Model file for the job. Use its own axes, mm. A direction names the side the tool comes from. Give positions to 0.01 mm unless a question says otherwise; leave off trailing zeros. Loops run counter-clockwise (first coordinate to the right, second up) from the corner with the lowest first, then second, coordinate; pieces in that order, holes last. Notation, with made-up numbers: M -30,21 L 10,21 A19 cw 10,33 Z; hole C 67,16.5 d4. An arc over 180 degrees is marked long. Answer in a Markdown table with one row per item.
```python
from build123d import *

# Parameters (mm, degrees)
F2_W      = 77
F2_H      = 64
F3_DEPTH  = 22
F4_W      = 73
F4_H      = 60
F5_DEPTH  = 20
F6_W      = 13
F6_H      = 12
F8_DEPTH  = 2
F7_W      = 12
F7_H      = 12
F9_DEPTH  = 2
F10_R     = 3.5
F11_DEPTH = 3


with BuildPart() as f3:
    # F2 (on Top) → F3 (new body)
    with BuildSketch(Plane.XY):
        with Locations((3.2737072408, 3.8249654726)):
            Rectangle(F2_W, F2_H)
    extrude(amount=F3_DEPTH)

    # F4 (on face) → F5 (cut)
    with BuildSketch(Plane.XY.offset(22)):
        with Locations((3.2737072408, 3.8249654726)):
            Rectangle(F4_W, F4_H)
    extrude(amount=-F5_DEPTH, mode=Mode.SUBTRACT)

    # F6 (on face) → F8 (cut)
    with BuildSketch(Plane.YZ.offset(41.7737072408)):
        with Locations((-9.3750345274, 12)):
            Rectangle(F6_W, F6_H)
    extrude(amount=-F8_DEPTH, mode=Mode.SUBTRACT)

    # F7 (on face) → F9 (cut)
    with BuildSketch(Plane.YZ.offset(41.7737072408)):
        with Locations((17.5249654726, 12)):
            Rectangle(F7_W, F7_H)
    extrude(amount=-F9_DEPTH, mode=Mode.SUBTRACT)

    # F10 (on face) → F11 (join)
    with BuildSketch(Plane.XY.offset(2)):
        with Locations((25.7737072408, -21.1750345274)):
            Circle(F10_R)
    extrude(amount=F11_DEPTH)


solid = f3.part
```
(1) Which spindle directions (+Z, -Z, +X, -X, +Y, -Y) get a long thin tool onto all of the face, cutting with end or side? Do faces 1 (the flat face through (41.774, 3, 11)), 2 (the flat face through (3, -26.175, 12)), 3 (the flat face through (41, -9, 6)). Say none if no direction does.
Established:
| item | result |
|---|---|
| face 1 | +Z, -Z, +X, +Y, -Y |
| face 2 | +Z |
| face 3 | +X |
(2) Saw through at D-D, the plane y = 1. Give the cut face in (x, z).
Established:
| item | result |
|---|---|
| outline | M -35.23,0 L 41.77,0 L 41.77,22 L 39.77,22 L 39.77,2 L -33.23,2 L -33.23,22 L -35.23,22 Z |
(3) Saw through at A-A, the plane y = 16. Give the cut face in (x, z).
Established:
| item | result |
|---|---|
| outline | M -35.23,0 L 41.77,0 L 41.77,6 L 39.77,6 L 39.77,2 L -33.23,2 L -33.23,22 L -35.23,22 Z; M 39.77,18 L 41.77,18 L 41.77,22 L 39.77,22 Z |
(4) Mould opens along Z. For faces 4 (the flat face through (-35.226, 3, 11)), 5 (the flat face through (26, -21, 5)), 6 (the flat face through (41, -2.875, 12)) say: pulls with the +Z half, pulls with the -Z half, needs draft (parallel to the pull), parting line crosses it, or undercut.
Established:
| item | result |
|---|---|
| face 4 | needs draft |
| face 5 | pulls with the +Z half |
| face 6 | undercut |
(5) Wall check: L1, parallel to X at y = -21, z = 4; L2, parallel to Y at x = 17, z = 12.25; L3, parallel to X at y = 29, z = 17.5. Give the ranges that are in metal, low to high.
Established:
| item | result |
|---|---|
| L1 | x = -35.23 to -33.23, 22.28 to 29.27, 39.77 to 41.77 |
| L2 | y = -28.18 to -26.18, 33.82 to 35.82 |
| L3 | x = -35.23 to -33.23, 39.77 to 41.77 |
(6) Saw through at B-B, the plane z = 13. Give the cut face in (x, y), and give its area (3 significant figures).
Established:
| item | result |
|---|---|
| outline | M -35.23,-28.18 L 41.77,-28.18 L 41.77,-15.88 L 39.77,-15.88 L 39.77,-26.18 L -33.23,-26.18 L -33.23,33.82 L 39.77,33.82 L 39.77,23.52 L 41.77,23.52 L 41.77,35.82 L -35.23,35.82 Z; M 39.77,-2.88 L 41.77,-2.88 L 41.77,11.52 L 39.77,11.52 Z |
| area | 498 mm2 |
(7) Saw through at C-C, the plane x = 10.5. Give the cut face in (y, z).
Established:
| item | result |
|---|---|
| outline | M -28.18,0 L 35.82,0 L 35.82,22 L 33.82,22 L 33.82,2 L -26.18,2 L -26.18,22 L -28.18,22 Z |
(8) Flat gauge pins, fed straight in: P1, Ø3, axis at x = 24.5, y = -21.5, coming from the +Z side; P2, Ø3, axis at x = 16.5, y = -0.5, coming from the +Z side. Where does each tip first touch, or does it go through?
Established:
| item | result |
|---|---|
| P1 | stops at z = 5 |
| P2 | stops at z = 2 |
